Check sheet for the modelled part. Datum: model origin and axes. Units: mm. A direction names the side the tool comes from. Round coordinates to 2 decimals unless told otherwise and drop trailing zeros. Order: outer loops, then holes, each group sorted by start corner. A loop starts at its lowest first (then second) coordinate and runs counter-clockwise, first axis right, second up.
(1) Tool access check on faces 1 (the flat face through (4.8, 2, 2.8)), 2 (the flat face through (3, 0, -3)). Record the directions out of +Z, -Z, +X, -X, +Y, -Y that give a thin tool (end or side, any length) a straight path to the whole face; none if there is none.
(2) Sectioned sample at A-A, the plane y = -29.5. Enter the section's corners in (x, z) (3 decimals), and give its area (3 significant figures).
(3) Thickness scan on probe 1 along Y at (x, z) = (-4.75, 1.75); probe 2 along X at (y, z) = (-73, -2.25); probe 3 along X at (y, z) = (-22, -1.5). Record the ranges inside material, lowest first.
(4) Depth check by flat-ended pin: pin 1 (5.5 mm diameter, centred on x = 3, z = -2, fed in from -Y); pin 2 (1 mm diameter, centred on y = -20, z = 0, fed in from +X) (3 decimals); pin 3 (1 mm diameter, centred on x = 4, y = -11, fed in from -Z); pin 4 (4 mm diameter, centred on x = -3, z = -4, fed in from -Y) (3 decimals). Enter the tip coordinate at first touch or a pass-through.
```python
from build123d import *

# Parameters (mm, degrees)
BOSS_EXTRUDE1_DEPTH = 3.9624
CUT_EXTRUDE1_DEPTH  = 0.0508


with BuildPart() as part:
    # Sketch1 → Boss-Extrude1 (new body)
    with BuildSketch(Plane(origin=(0, 0, 0), x_dir=(1, 0, 0), z_dir=(0, 1, 0))):
        Polygon((6.415804866, 0), (3.207902433, 5.55625), (-3.207902433, 5.55625), (-6.415804866, 0), (-3.207902433, -5.55625), (3.207902433, -5.55625), align=None)
    extrude(amount=BOSS_EXTRUDE1_DEPTH)

    # Sketch2 → Cut-Revolve1 (revolve, cut)
    with BuildSketch(Plane.XY):
        Polygon((5.55625, 3.9624), (6.415804866, 3.4544), (6.415804866, 3.9624), align=None)
    revolve(axis=Axis((0, 0, 0), (0, 1, 0)), mode=Mode.SUBTRACT)

    # Sketch3 → Cut-Extrude1 (cut)
    with BuildSketch(Plane(origin=(0, 3.9624, 0), x_dir=(-1, 0, 0), z_dir=(0, -1, 0))):
        with BuildLine():
            Line((0.127, 4.7625), (0.127, 2.7305))
            ThreePointArc((0.127, 2.7305), (0, 2.6035), (-0.127, 2.7305))
            Line((-0.127, 2.7305), (-0.127, 4.7625))
            ThreePointArc((-0.127, 4.7625), (0, 4.8895), (0.127, 4.7625))
        make_face()
        with BuildLine():
            Line((4.060945986, -2.491235226), (2.301182365, -1.475235226))
            ThreePointArc((2.301182365, -1.475235226), (2.254697139, -1.30175), (2.428182365, -1.255264774))
            Line((2.428182365, -1.255264774), (4.187945986, -2.271264774))
            ThreePointArc((4.187945986, -2.271264774), (4.234431212, -2.44475), (4.060945986, -2.491235226))
        make_face()
        with BuildLine():
            Line((-4.187945986, -2.271264774), (-2.428182365, -1.255264774))
            ThreePointArc((-2.428182365, -1.255264774), (-2.254697139, -1.30175), (-2.301182365, -1.475235226))
            Line((-2.301182365, -1.475235226), (-4.060945986, -2.491235226))
            ThreePointArc((-4.060945986, -2.491235226), (-4.234431212, -2.44475), (-4.187945986, -2.271264774))
        make_face()
    extrude(amount=CUT_EXTRUDE1_DEPTH, mode=Mode.SUBTRACT)

    # Bolt Length Sketch → Bolt Length (revolve)
    with BuildSketch(Plane.XY, mode=Mode.PRIVATE) as bolt_length_sk:
        Polygon((0, 0), (0, -88.9), (2.778125, -88.9), (3.175, -88.265), (3.175, 0), align=None)
    revolve(bolt_length_sk.sketch.rotate(Axis((0, 0, 0), (0, -1, 0)), 180), axis=Axis((0, 0, 0), (0, -1, 0)))


solid = part.part
```
Derived:
1. face 1: +Z, +X, +Y, -Y
1. face 2: -Y
2. outline: circle Ø6.35 at (0, 0)
2. area: 31.7 mm2
3. probe 1: y = 0 to 3.96
3. probe 2: x = -2.24 to 2.24
3. probe 3: x = -2.8 to 2.8
4. pin 1: stops at y = -88.9
4. pin 2: stops at x = 3.175
4. pin 3: passes through
4. pin 4: stops at y = -88.545
